Work out the finished part from the listing and answer in its coordinate system (mm). Coordinates: 2 decimals unless noted, no trailing zeros. Use a Markdown table: item, result. Add a question column.
(1) For a pull along Z with two mould halves and no side action, classify faces 1 (the face through (-69, 0, -69)), 2 (the face through (-69, 1, 0)), 3 (the face through (-138, 1, -138)), 4 (the face through (-59, 1, -23)) as released by +Z, released by -Z, zero draft, split by the parting line, or undercut.
(2) Given pin 1 Ø1.8 at (x, z) = (-82.5, -23) entering from -Y, flat-ended and moving along its own axis, determine where the tip first touches the part or whether it passes through.
(3) Find the intervals of material crossed by line 1 (Z direction, x = -57.5, y = 1.8), in increasing order. Write a range as from..to.
Autodesk Inventor part; units mm, degrees
ref_plane "YZ Plane" through (0, 0, 0) normal (1, 0, 0) x (0, 1, 0)
ref_plane "XZ Plane" through (0, 0, 0) normal (0, 1, 0) x (-1, 0, 0)
ref_plane "XY Plane" through (0, 0, 0) normal (0, 0, 1) x (1, 0, 0)
sketch "Sketch1" plane through (0, 0, 0) normal (0, 1, 0) x (-1, 0, 0)
  line L0 (0, 0) -> (140, 0)
  line L1 (140, 0) -> (140, -140)
  line L2 (140, -140) -> (0, -140)
  line L3 (0, -140) -> (0, 0)
  circle A0 centre (82.5, -23) radius 1.5
  circle A1 centre (57.5, -23) radius 1.5
  line L4 (82.5, -23) -> (57.5, -23) construction
  point P0 (70, -23)
  point P1 (70, 0)
  dimension "d0" = 140
  dimension "d1" = 140
  dimension "d2" = 3
  dimension "d3" = 23
  dimension "d4" = 25
extrude "Extrusion1" add sketch "Sketch1" along normal blind 3
chamfer "Chamfer1" distance 4 angle 45 4 edges at (-140, 1.5, 0) (-140, 1.5, -140) (0, 1.5, -140) (0, 1.5, 0)
properties part number "table"
Model answer:
| question | item | result |
|---|---|---|
| 1 | face 1 | zero draft |
| 1 | face 2 | released by +Z |
| 1 | face 3 | released by -Z |
| 1 | face 4 | undercut |
| 2 | pin 1 | through |
| 3 | line 1 | -140..-24.5, -21.5..0 |
